from build123d import *

# Parameters (mm, degrees)
F1_DEPTH = 30
F2_R     = 10


with BuildPart() as f1:
    # F0 (on Front) → F1 (new body)
    with BuildSketch(Plane.XZ):
        Polygon((0, 10), (0, 0), (80, 0), (80, 10), (29.95, 10), (29.95, 20), (35.5, 20), (35.5, 26.7), (44.5, 26.7), (44.5, 40), (19.5, 40), (19.5, 10), align=None)
    extrude(amount=F1_DEPTH)

    # F2
    f2_edges = [f1.edges().sort_by_distance(p)[0] for p in [
        (19.5, -15, 10),
        (19.5, -15, 40),
    ]]
    fillet(f2_edges, radius=F2_R)


solid = f1.part
The model under review builds one solid part; all positions refer to its coordinate system, in mm. A direction names the side the tool comes from. Round coordinates to 2 decimals unless told otherwise and drop trailing zeros. Loops run counter-clockwise (first coordinate to the right, second up) from the corner with the lowest first, then second, coordinate; pieces in that order, holes last. Notation, with made-up numbers: (-13, 50) -> (0, 50) arc R17 cw to (0, 56) -> close; hole circle Ø3 at (29.25, 32). An arc over 180 degrees is marked (long way). Write item = value, one per line. Start each with the question number.
Item 1: Mouldability with a two-part tool opening along Z and no side actions: class faces 1 (the flat face through (29.95, -15, 15)), 2 (the flat face through (37, -15, 40)), 3 (the flat face through (44.5, -15, 33)) as released by +Z, released by -Z, zero draft, split by the parting line, or undercut.
Item 2: Take a section at C-C on x = 45.5. Give the boundary of the cut face in (y, z), plus the area to 3 significant figures.
Item 3: Take a section at B-B on z = 23.5. Give the boundary of the cut face in (x, y), plus the area to 3 significant figures.
Item 4: To check wall thickness, follow L1, parallel to Z at x = 41.5, y = -2.5; L2, parallel to X at y = -8.75, z = 20.5; L3, parallel to X at y = -14.5, z = 30.5. State the ranges of each line that lie inside material, in increasing order.
Item 5: For faces 4 (the flat face through (0, -15, 5)), 5 (the flat face through (33, -15, 20)), 6 (the flat face through (19.5, -15, 25)), list the 3-axis set-ups (+Z, -Z, +X, -X, +Y, -Y) from which the entire face can be reached by the end or side of a thin tool; tool diameter is ignored.
Item 6: Insertion check: pin 1 (6 mm diameter, centred on x = 10.5, y = -6, fed in from +Z); pin 2 (2 mm diameter, centred on x = 68.5, y = -11, fed in from -Z); pin 3 (10.5 mm diameter, centred on x = 3, y = -11.5, fed in from +Z); pin 4 (6.5 mm diameter, centred on y = -18, z = 31.5, fed in from +X). Each pin has a flat end and moves straight along its axis. Give the tip position at first contact, or say it passes through.
Item 7: Take a section at A-A on y = -2.25. Give the boundary of the cut face in (x, z), plus the area to 3 significant figures.
Result:
q1.face_1 = undercut
q1.face_2 = released by +Z
q1.face_3 = zero draft
q2.outline = (-30, 0) -> (0, 0) -> (0, 10) -> (-30, 10) -> close
q2.area = 300 mm²
q3.outline = (19.5, -30) -> (35.5, -30) -> (35.5, 0) -> (19.5, 0) -> close
q3.area = 480 mm²
q4.L1 = 0 to 10, 26.7 to 40
q4.L2 = 19.5 to 35.5
q4.L3 = 19.51 to 44.5
q5.face_4 = +Z, -Z, -X, +Y, -Y
q5.face_5 = +X, +Y, -Y
q5.face_6 = +Z, -X, +Y, -Y
q6.pin_1 = 10.83
q6.pin_2 = 0
q6.pin_3 = 10
q6.pin_4 = 44.5
q7.outline = (0, 0) -> (80, 0) -> (80, 10) -> (29.95, 10) -> (29.95, 20) -> (35.5, 20) -> (35.5, 26.7) -> (44.5, 26.7) -> (44.5, 40) -> (29.5, 40) arc R10 ccw to (19.5, 30) -> (19.5, 20) arc R10 cw to (9.5, 10) -> (0, 10) -> close
q7.area = 1,340 mm²
